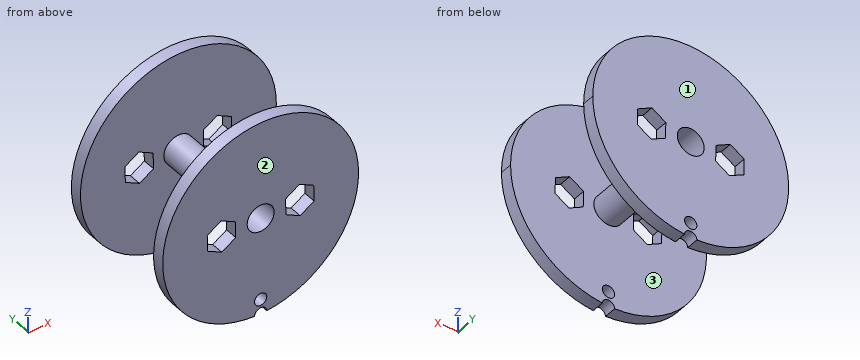
```python
from build123d import *

# Parameters (mm, degrees)
SKETCH1_R           = 20
SKETCH1_R_2         = 2.75
BOSS_EXTRUDE1_DEPTH = 2.5
CUT_EXTRUDE3_DEPTH  = 2.5
SKETCH4_R           = 1.25
CUT_EXTRUDE4_DEPTH  = 5
SKETCH2_R           = 3
SKETCH2_R_2         = 2.75
BOSS_EXTRUDE2_DEPTH = 10


with BuildPart() as part:
    # Sketch1 → Boss-Extrude1 (new body)
    with BuildSketch(Plane(origin=(0, 0, 0), x_dir=(1, 0, 0), z_dir=(0, 1, 0))):
        Circle(SKETCH1_R)
        Circle(SKETCH1_R_2, mode=Mode.SUBTRACT)
    extrude(amount=BOSS_EXTRUDE1_DEPTH)

    # Sketch3 → Cut-Extrude3 (cut)
    with BuildSketch(Plane.XZ):
        Polygon((-5.161329605, 1.721273866), (-8.071331697, 3.318997608), (-10.910002092, 1.597723742), (-10.838670395, -1.721273866), (-7.928668303, -3.318997608), (-5.089997908, -1.597723742), align=None)
        Polygon((5.161329605, -1.721273866), (8.071331697, -3.318997608), (10.910002092, -1.597723742), (10.838670395, 1.721273866), (7.928668303, 3.318997608), (5.089997908, 1.597723742), align=None)
    extrude(amount=-CUT_EXTRUDE3_DEPTH, mode=Mode.SUBTRACT)

    # Sketch4 → Cut-Extrude4 (cut)
    with BuildSketch(Plane(origin=(0, 2.5, 0), x_dir=(1, 0, 0), z_dir=(0, 1, 0))):
        with Locations((0, 17)):
            Circle(SKETCH4_R)
        with Locations((0, 20)):
            Circle(SKETCH4_R)
    extrude(amount=-CUT_EXTRUDE4_DEPTH, mode=Mode.SUBTRACT)

    # Sketch2 → Boss-Extrude2 (add)
    with BuildSketch(Plane(origin=(0, 2.5, 0), x_dir=(1, 0, 0), z_dir=(0, 1, 0))):
        Circle(SKETCH2_R)
        Circle(SKETCH2_R_2, mode=Mode.SUBTRACT)
    extrude(amount=BOSS_EXTRUDE2_DEPTH)

    # Mirror7: part across plane


with BuildPart() as part_1:
    add(part.part)
    add(part.part.mirror(Plane.ZX.offset(12.5)))


solid = part_1.part
```
Part model, mm, in its own coordinate system. Face numbers are marked on the shaded views. Coordinates: 2 decimals unless noted, no trailing zeros. Order: outer loops, then holes, each group sorted by start corner. A loop starts at its lowest first (then second) coordinate and runs counter-clockwise, first axis right, second up. Notation, with made-up numbers: (73.25, 25) - (94.25, 25) arc R16 ccw to (94.25, 53) - close; hole circle Ø6 at (40.5, 2). An arc over 180 degrees is marked (long way). Return JSON: item names as keys, results as strings. Group by question number.
Item 1: Cut at B-B (x = 12). List the corners of the cut face in (y, z).
Item 2: Cut at D-D (y = 3.75). List the corners of the cut face in (x, z), plus the area to 3 significant figures.
Item 3: Cut at C-C (z = -5.5). List the corners of the cut face in (x, y), plus the area to 3 significant figures.
Item 4: Pin check, flat tips, straight feed: pin 1 (1 mm diameter, centred on x = 3, y = 3.5, fed in from -Z); pin 2 (1.5 mm diameter, centred on x = 3.5, y = 11.5, fed in from -Z); pin 3 (3 mm diameter, centred on y = 22.5, z = -14.5, fed in from +X). Stop position of each tip, or through.
Item 5: Drill centre lines: probe 1 along Z at (x, y) = (0, 1.3); probe 2 along Y at (x, z) = (-7, 5); probe 3 along X at (y, z) = (4.75, 0). Where is each one in solid material? Low to high. Write a range as from..to.
Item 6: Pull direction Y, two halves, no side cores. Call the marked faces 1, 2 and 3: pulls with the +Y half, pulls with the -Y half, needs draft (parallel to the pull), parting line crosses it, or undercut.
Item 7: Cut at A-A (x = 0). List the corners of the cut face in (y, z).
Check values:
{
 "1": {"outline": "(0, -16) - (2.5, -16) - (2.5, 16) - (0, 16) - close; (22.5, -16) - (25, -16) - (25, 16) - (22.5, 16) - close"},
 "2": {"outline": "circle Ø6 at (0, 0); hole circle Ø5.5 at (0, 0)", "area": "4.52 mm2"},
 "3": {"outline": "(-19.23, 0) - (19.23, 0) - (19.23, 2.5) - (-19.23, 2.5) - close; (-19.23, 22.5) - (19.23, 22.5) - (19.23, 25) - (-19.23, 25) - close", "area": "192 mm2"},
 "4": {"pin 1": "stops at z = -1.66", "pin 2": "stops at z = -1.2", "pin 3": "stops at x = 15.2"},
 "5": {"probe 1": "z = -18.75..-18.25, -15.75..-2.75, 2.75..20", "probe 2": "y = 0..2.5, 22.5..25", "probe 3": "x = -3..-2.75, 2.75..3"},
 "6": {"face 1": "pulls with the +Y half", "face 2": "pulls with the -Y half", "face 3": "undercut"},
 "7": {"outline": "(0, -18.75) - (2.5, -18.75) - (2.5, -18.25) - (0, -18.25) - close; (0, -15.75) - (2.5, -15.75) - (2.5, -3) - (22.5, -3) - (22.5, -15.75) - (25, -15.75) - (25, -2.75) - (0, -2.75) - close; (0, 2.75) - (25, 2.75) - (25, 20) - (22.5, 20) - (22.5, 3) - (2.5, 3) - (2.5, 20) - (0, 20) - close; (22.5, -18.75) - (25, -18.75) - (25, -18.25) - (22.5, -18.25) - close"}
}
